Input: part model. Units: mm. Frame: model coordinates. A direction names the side the tool comes from. Give positions to 0.01 mm unless a question says otherwise; leave off trailing zeros. Order: outer loops, then holes, each group sorted by start corner. A loop starts at its lowest first (then second) coordinate and runs counter-clockwise, first axis right, second up. Notation, with made-up numbers: (-25, 6.25) - (-7, 6.25) arc R9 ccw to (-7, 12.25) - close; hole circle Ø11 at (-5.5, -17.5). An arc over 180 degrees is marked (long way). Use a Markdown table: item, result.
from build123d import *

# Parameters (mm, degrees)
BOSS_EXTRUDE1_DEPTH     = 13
CUT_EXTRUDE1_DEPTH      = 32.130049791
CUT_EXTRUDE1_DEPTH_BACK = 32.130049791
SKETCH2_W               = 11.385886766
SKETCH2_H               = 3


with BuildPart() as part:
    # Sketch1 → Boss-Extrude1 (new body)
    with BuildSketch(Plane(origin=(0, 0, 0), x_dir=(1, 0, 0), z_dir=(0, 1, 0))):
        Polygon((2.453447834, -5.3), (-2.546552166, -5.3), (-2.546552166, -18.3), (-10.746552166, -18.3), (-10.746552166, -5.3), (-15.746552166, -5.3), (-15.746552166, 0), (-13.293104332, 0), (-13.293104332, 0.9), (-16.746552166, 0.9), (-16.746552166, -6.8), (-11.746552166, -6.8), (-11.746552166, -19.8), (-1.546552166, -19.8), (-1.546552166, -6.8), (3.453447834, -6.8), (3.453447834, 0.9), (0, 0.9), (0, 0), (2.453447834, 0), align=None)
    extrude(amount=BOSS_EXTRUDE1_DEPTH)

    # Sketch2 → Cut-Extrude1 (cut, two sides: drawn at the far end of the back side and taken through both)
    with BuildSketch(Plane.ZY.offset(16.746552166).offset(-CUT_EXTRUDE1_DEPTH_BACK)):
        with Locations((4.792943383, 1.5)):
            Rectangle(SKETCH2_W, SKETCH2_H)
    extrude(amount=CUT_EXTRUDE1_DEPTH + CUT_EXTRUDE1_DEPTH_BACK, mode=Mode.SUBTRACT)


solid = part.part
1. Set-up query: faces 1 (the face through (1, 8, 0)), 2 (the face through (-10.747, 6, 12)), 3 (the face through (-11.747, 6, 13)), 4 (the face through (-11, 1, 10.486)). Return all of +Z, -Z, +X, -X, +Y, -Y with unobstructed straight access to the full face (end or side cutting, diameter ignored); none if empty.
Response:
| item | result |
|---|---|
| face 1 | +Y, -Y |
| face 2 | -Z, +Y, -Y |
| face 3 | +Z, -X, +Y, -Y |
| face 4 | -Z, +X, -X, -Y |
2. Section query B-B (y = 2). Return loops of the section in (x, z).
Response:
| item | result |
|---|---|
| outline | (-11.75, 10.49) - (-10.75, 10.49) - (-10.75, 18.3) - (-2.55, 18.3) - (-2.55, 10.49) - (-1.55, 10.49) - (-1.55, 19.8) - (-11.75, 19.8) - close |
3. Section query A-A (z = 1.75). Return loops of the section in (x, y).
Response:
| item | result |
|---|---|
| outline | (-16.75, 3) - (-15.75, 3) - (-15.75, 13) - (-16.75, 13) - close; (2.45, 3) - (3.45, 3) - (3.45, 13) - (2.45, 13) - close |
4. Material intervals for line 1 along X through (y, z) = (4.75, 12); line 2 along Z through (x, y) = (-14.75, 8.25); line 3 along X through (y, z) = (8.75, 6.75), sorted ascending.
Response:
| item | result |
|---|---|
| line 1 | x = -11.75 to -10.75, -2.55 to -1.55 |
| line 2 | z = -0.9 to 0, 5.3 to 6.8 |
| line 3 | x = -16.75 to -10.75, -2.55 to 3.45 |
5. Section query C-C (z = 6.5). Return loops of the section in (x, y), then the cut area to 3 significant figures.
Response:
| item | result |
|---|---|
| outline | (-16.75, 3) - (-10.75, 3) - (-10.75, 13) - (-16.75, 13) - close; (-2.55, 3) - (3.45, 3) - (3.45, 13) - (-2.55, 13) - close |
| area | 120 mm^2 |
6. Pin query (flat end, axial travel): pin 1 (4 mm diameter, centred on x = 1.5, z = 15, fed in from -Y); pin 2 (6.5 mm diameter, centred on x = -7, y = 5, fed in from -Z); pin 3 (0.5 mm diameter, centred on x = -11, y = 1.5, fed in from -Z); pin 4 (1.5 mm diameter, centred on x = -13, y = 9, fed in from +Z). Return the tip coordinate at first contact, or that it passes through.
Response:
| item | result |
|---|---|
| pin 1 | passes through |
| pin 2 | stops at z = 18.3 |
| pin 3 | stops at z = 10.49 |
| pin 4 | stops at z = 6.8 |
7. Section query D-D (x = -7.25). Return loops of the section in (y, z), then the cut area to 3 significant figures.
Response:
| item | result |
|---|---|
| outline | (0, 18.3) - (13, 18.3) - (13, 19.8) - (0, 19.8) - close |
| area | 19.5 mm^2 |
